Model file for the job. Use its own axes, mm. A direction names the side the tool comes from. Round coordinates to 2 decimals unless told otherwise and drop trailing zeros. Loops run counter-clockwise (first coordinate to the right, second up) from the corner with the lowest first, then second, coordinate; pieces in that order, holes last. Notation, with made-up numbers: M -37.75,49.25 L 9.25,49.25 A21 cw 9.25,80.25 Z; hole C -3,33.5 d5. An arc over 180 degrees is marked long. Use a Markdown table: item, result. Add a question column.
Q1. Cut at B-B (y = 2.15). State how many separate pieces and enclosed holes the cut face has, plus the area to 3 significant figures.
Q2. Tool access for faces 4 (the face through (-164.776, 1.521, 36.626)), 5 (the face through (-115.25, 1.48, -11.03)), 6 (the face through (-204, 1.6, -26)): list every direction of +Z, -Z, +X, -X, +Y, -Y with a clear straight run to the whole face (end or side of a thin tool).
Q3. Cut at A-A (z = 31). Give the cut face in (x, y), plus the area to 3 significant figures.
Q4. Mould opens along Z. For faces 1 (the face through (-164.776, 1.521, 16.362)), 2 (the face through (-159, 1, -36.006)), 3 (the face through (-157, 3, 26)) say: +Z half, -Z half, draft (parallel to the pull), parting line (faces both ways), or undercut.
Q5. Pin check, flat tips, straight feed: pin 1 (8 mm diameter, centred on x = -112.77, z = 76.49, fed in from -Y); pin 2 (4.5 mm diameter, centred on x = -202.77, z = -23.51, fed in from +Y); pin 3 (1 mm diameter, centred on y = 2, z = 4, fed in from -X). Stop position of each tip, or through.
Q6. Probe line 1 (X direction, y = 1.5, z = -28); line 2 (X direction, y = 0.3, z = 15); line 3 (Y direction, x = -116, z = 75). List the from-to ranges inside material, lowest first. Write a range as from..to.
from build123d import *

# Parameters (mm, degrees)
F1_DEPTH       = 3
F2_D           = 6
F2_DEPTH       = 34.5
F3_D           = 5.1
F3_DEPTH       = 34.5
F3_CBORE_D     = 10.2
F3_CBORE_DEPTH = 1.6
F5_D           = 5.1
F5_DEPTH       = 34.5
F5_CBORE_D     = 10.2
F5_CBORE_DEPTH = 1.6


with BuildPart() as f1:
    # F0 (on Front) → F1 (new body)
    with BuildSketch(Plane.XZ):
        with BuildLine():
            Line((-157.773511, 88.993683), (-210.773511, 88.993683))
            ThreePointArc((-210.773511, 88.993683), (-212.187724, 88.407897), (-212.773511, 86.993683))
            Line((-212.773511, 86.993683), (-212.773511, 68.493683))
            ThreePointArc((-212.773511, 68.493683), (-212.187724, 67.07947), (-210.773511, 66.493683))
            Line((-210.773511, 66.493683), (-203.519511, 66.493683))
            ThreePointArc((-203.519511, 66.493683), (-202.830681, 66.356667), (-202.246719, 65.966476))
            Line((-202.246719, 65.966476), (-198.300719, 62.020476))
            ThreePointArc((-198.300719, 62.020476), (-197.910528, 61.436514), (-197.773511, 60.747683))
            Line((-197.773511, 60.747683), (-197.773511, 26.493683))
            Line((-197.773511, 26.493683), (-157.773511, 26.493683))
            Line((-157.773511, 26.493683), (-157.773511, 88.993683))
        make_face()
    extrude(amount=-F1_DEPTH)

    # F2
    with Locations(Plane.XZ):
        with Locations((-187.773511, 56.493683), (-167.773511, 56.493683), (-167.773511, 36.493683)):
            Hole(F2_D / 2, depth=F2_DEPTH)

    # F3
    with Locations(Plane.XZ):
        with Locations((-202.773511, 76.493683)):
            CounterBoreHole(F3_D / 2, F3_CBORE_D / 2, F3_CBORE_DEPTH, depth=F3_DEPTH)

    # F4: F1 across face


with BuildPart() as f1_1:
    add(f1.part)
    add(f1.part.mirror(Plane(origin=(-157.773511, 1.5, 57.743683), x_dir=(0, 1, 0), z_dir=(1, 0, 0))))

    # F5
    with Locations(Plane.XZ):
        with Locations((-157.773511, 76.493683)):
            CounterBoreHole(F5_D / 2, F5_CBORE_D / 2, F5_CBORE_DEPTH, depth=F5_DEPTH)

    # F6: F1 across face


with BuildPart() as f1_2:
    add(f1_1.part)
    add(f1_1.part.mirror(Plane(origin=(-157.773511, 1.5, 26.493683), x_dir=(1, 0, 0), z_dir=(0, 0, -1))))


solid = f1_2.part
Checked values:
| question | item | result |
|---|---|---|
| 1 | separate pieces | 1 |
| 1 | enclosed holes | 18 |
| 1 | area | 10,900 mm^2 |
| 2 | face 4 | +Y, -Y |
| 2 | face 5 | +X, +Y, -Y |
| 2 | face 6 | -Y |
| 3 | outline | M -197.77,0 L -117.77,0 L -117.77,3 L -197.77,3 Z |
| 3 | area | 240 mm^2 |
| 4 | face 1 | undercut |
| 4 | face 2 | -Z half |
| 4 | face 3 | draft |
| 5 | pin 1 | stops at y = 1.6 |
| 5 | pin 2 | passes through |
| 5 | pin 3 | stops at x = -197.77 |
| 6 | line 1 | x = -212.77..-205.19, -200.36..-160.19, -155.36..-115.19, -110.36..-102.77 |
| 6 | line 2 | x = -197.77..-170.38, -165.17..-150.38, -145.17..-117.77 |
| 6 | line 3 | y = 1.6..3 |
